```python
from build123d import *

# Parameters (mm, degrees)
EXTRUDE_1_DEPTH              = 2.4
SKETCH_2_R                   = 2.75
EXTRUDE_3_DEPTH              = 3.9
FILLET_1_R                   = 1
FILLET_2_R                   = 0.2
HOLE_WIZARD_M3_1_D           = 2.5
HOLE_WIZARD_M3_1_DEPTH       = 7.5
HOLE_WIZARD_M3_1_CSINK_D     = 3.05
HOLE_WIZARD_M3_1_CSINK_ANGLE = 90
HOLE_WIZARD_M3_1_TIP         = 0.751075774


with BuildPart() as part:
    # 草图1 → 凸台-拉伸1 (new body)
    with BuildSketch(Plane.XY):
        Polygon((2.409913138, -2.067764977), (2.995693568, 1.05316351), (0.58578043, 3.120928487), (-2.409913138, 2.067764977), (-2.995693568, -1.05316351), (-0.58578043, -3.120928487), align=None)
    extrude(amount=EXTRUDE_1_DEPTH)

    # 草图2 → 凸台-拉伸3 (add)
    with BuildSketch(Plane.XY.offset(2.4)):
        Circle(SKETCH_2_R)
    extrude(amount=-EXTRUDE_3_DEPTH)

    # 圆角1
    fillet_1_edges = [part.edges().sort_by_distance(p)[0] for p in [
        (-2.75, 0, -1.5),
    ]]
    fillet(fillet_1_edges, radius=FILLET_1_R)

    # 圆角2
    fillet_2_edges = [part.edges().sort_by_distance(p)[0] for p in [
        (-0.58578043, -3.120928487, 1.2),
        (-2.995693568, -1.05316351, 1.2),
        (-2.409913138, 2.067764977, 1.2),
        (0.58578043, 3.120928487, 1.2),
        (2.995693568, 1.05316351, 1.2),
        (2.409913138, -2.067764977, 1.2),
    ]]
    fillet(fillet_2_edges, radius=FILLET_2_R)

    # M3 螺纹孔1
    with Locations(Plane.XY.offset(2.4)):
        with Locations((0, 0)):
            CounterSinkHole(HOLE_WIZARD_M3_1_D / 2, HOLE_WIZARD_M3_1_CSINK_D / 2, depth=HOLE_WIZARD_M3_1_DEPTH, counter_sink_angle=HOLE_WIZARD_M3_1_CSINK_ANGLE)
            with Locations((0, 0, -(HOLE_WIZARD_M3_1_DEPTH + HOLE_WIZARD_M3_1_TIP / 2))):  # 118° drill point
                Cone(0, HOLE_WIZARD_M3_1_D / 2, HOLE_WIZARD_M3_1_TIP, mode=Mode.SUBTRACT)


solid = part.part
```
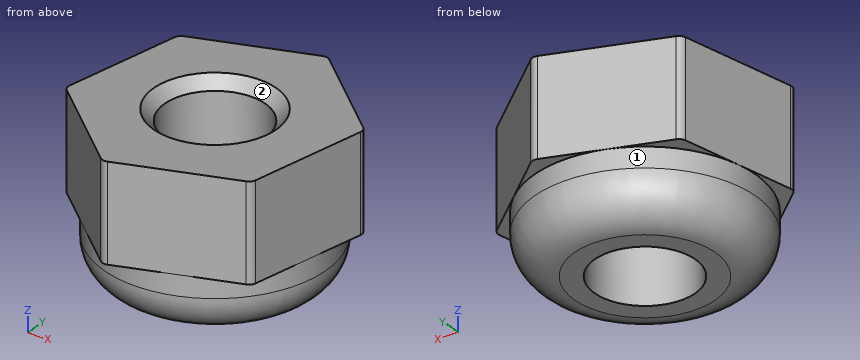
Input: part model. Units: mm. Frame: model coordinates. Face numbers are marked on the shaded views. A direction names the side the tool comes from. Coordinates: 2 decimals unless noted, no trailing zeros. Write each loop counter-clockwise with the first axis right and the second up, starting at its lowest first coordinate (ties: lowest second). Pieces come first, ordered by that corner, then holes. Notation, with made-up numbers: M 48.25,54.25 L 105.25,54.25 A23 ccw 105.25,74.25 Z; hole C 89,74 d2. An arc over 180 degrees is marked long. Use one line per item in the form item = value.
Q1. Section B-B (x = 0). Return loops of the section in (y, z) (3 decimals), plus the area to 3 significant figures.
Answer below:
outline = M -2.915,0 L -2.75,0 L -2.75,-0.5 A1 ccw -1.75,-1.5 L -1.25,-1.5 L -1.25,2.125 L -1.525,2.4 L -2.915,2.4 Z; M 1.25,-1.5 L 1.75,-1.5 A1 ccw 2.75,-0.5 L 2.75,0 L 2.915,0 L 2.915,2.4 L 1.525,2.4 L 1.25,2.125 Z
area = 12.0 mm²
Q2. Material intervals for probe 1 along Y at (x, z) = (0, 0.45) (3 decimals); probe 2 along X at (y, z) = (0, -0.1); probe 3 along Z at (x, y) = (-1.3, 1.25), sorted ascending. Write a range as from..to.
Answer below:
probe_1 = -2.915..-1.25, 1.25..2.915
probe_2 = -2.75..-1.25, 1.25..2.75
probe_3 = -1.5..2.4
Q3. Section C-C (y = 0). Return loops of the section in (x, z) (3 decimals), plus the area to 3 significant figures.
Answer below:
outline = M -2.798,0 L -2.75,0 L -2.75,-0.5 A1 ccw -1.75,-1.5 L -1.25,-1.5 L -1.25,2.125 L -1.525,2.4 L -2.798,2.4 Z; M 1.25,-1.5 L 1.75,-1.5 A1 ccw 2.75,-0.5 L 2.75,0 L 2.798,0 L 2.798,2.4 L 1.525,2.4 L 1.25,2.125 Z
area = 11.4 mm²
Q4. Section D-D (z = -0.9). Return loops of the section in (x, y), plus the area to 3 significant figures.
Answer below:
outline = C 0,0 d5.33; hole C 0,0 d2.5
area = 17.4 mm²
Q5. Set-up query: the marked faces 1 and 2. Return all of +Z, -Z, +X, -X, +Y, -Y with unobstructed straight access to the full face (end or side cutting, diameter ignored); none if empty.
Answer below:
face_1 = -Z
face_2 = +Z
Q6. First-contact query: pin 1 (1.1 mm diameter, centred on x = -0.5, y = -3, fed in from -Z); pin 2 (0.5 mm diameter, centred on x = 0.5, y = 2.5, fed in from -Z). Flat tips, straight axial feed; report the tip coordinate or a pass-through.
Answer below:
pin_1 = -1.17
pin_2 = -1.34
Q7. Section A-A (z = 0.2). Return loops of the section in (x, y), plus the area to 3 significant figures.
Answer below:
outline = M -2.97,-0.94 A0.2 ccw -2.91,-1.13 L -0.67,-3.05 A0.2 ccw -0.48,-3.08 L 2.3,-2.11 A0.2 ccw 2.43,-1.95 L 2.97,0.94 A0.2 ccw 2.91,1.13 L 0.67,3.05 A0.2 ccw 0.48,3.08 L -2.3,2.11 A0.2 ccw -2.43,1.95 Z; hole C 0,0 d2.5
area = 21.3 mm²
